The model under review builds one solid part; all positions refer to its coordinate system, in mm. Face numbers are marked on the shaded views. A direction names the side the tool comes from. Give positions to 0.01 mm unless a question says otherwise; leave off trailing zeros. Write each loop counter-clockwise with the first axis right and the second up, starting at its lowest first coordinate (ties: lowest second). Pieces come first, ordered by that corner, then holes. Notation, with made-up numbers: M -13.5,-36.75 L 27.5,-36.75 A10 cw 27.5,-18.75 Z; hole C 65,40.5 d9. An arc over 180 degrees is marked long. Write item = value, one per line. Start each with the question number.
Autodesk Inventor part; units mm, degrees
ref_plane "YZ Plane" through (0, 0, 0) normal (1, 0, 0) x (0, 1, 0)
ref_plane "XZ Plane" through (0, 0, 0) normal (0, 1, 0) x (-1, 0, 0)
ref_plane "XY Plane" through (0, 0, 0) normal (0, 0, 1) x (1, 0, 0)
sketch "スケッチ1" plane through (0, 0, 0) normal (0, 0, 1) x (1, 0, 0)
  line L0 (-32.5, -17.075) -> (32.5, -17.075)
  line L1 (32.5, -17.075) -> (32.5, 17.075)
  line L2 (32.5, 17.075) -> (-32.5, 17.075)
  line L3 (-32.5, 17.075) -> (-32.5, -17.075)
  line L4 (-32.5, -17.075) -> (32.5, 17.075) construction
  line L5 (32.5, -17.075) -> (-32.5, 17.075) construction
  point P0 (0, 0)
  dimension "d0" = 65
  dimension "d1" = 34.15
ref_plane "作業平面2" through (0, 0, -11.7) normal (0, 0, -1) x (-1, 0, 0)
ref_plane "作業平面1" through (35.75, -19.2175, -13.7) normal (0, 1, 0) x (-1, 0, 0)
sketch "スケッチ3" plane through (35.75, -19.2175, -13.7) normal (0, 1, 0) x (-1, 0, 0)
  line L0 (71.5, 0) -> (0, 0)
  line L1 (0, 0) -> (71.5, 0)
  line L2 (71.5, 0) -> (71.5, 20)
  line L3 (71.5, 20) -> (0, 20)
  line L4 (0, 20) -> (0, 0)
  line L5 (71.5, 1) -> (0, 1)
  point P0 (35.75, 13.7)
  dimension "d6" = 20
  dimension "d10" = 1
extrude "押し出し3" add sketch "スケッチ3" against normal blind 2
sketch "スケッチ4" plane through (35.75, -19.2175, -13.7) normal (0, 1, 0) x (1, 0, 0)
  line L0 (0, 0) -> (-71.5, 0)
  line L1 (0, -1) -> (-71.5, -1)
  line L2 (0, 0) -> (-71.5, 0)
  line L3 (-71.5, 0) -> (-71.5, -1)
  line L4 (-71.5, -1) -> (0, -1)
  line L5 (0, -1) -> (0, 0)
  point P0 (-35.75, -13.7)
extrude "押し出し4" add sketch "スケッチ4" along normal blind 38
sketch "スケッチ5" plane through (35.75, -19.2175, -13.7) normal (0, 1, 0) x (1, 0, 0)
  line L0 (0, 0) -> (0, -20)
  line L1 (0, -10) -> (-71.5, -10.5)
  line L2 (-71.5, -1) -> (-71.5, -20)
  point P0 (-35.75, -13.7)
  point P1 (-7, -10.049)
  point P2 (-20, -10.1399)
  point P3 (-33, -10.2308)
  point P4 (-46, -10.3217)
  point P5 (-59, -10.4126)
  dimension "d13" = 71.5
  dimension "d14" = 7
  dimension "d15" = 13
  dimension "d16" = 13
  dimension "d17" = 13
  dimension "d18" = 13
hole "穴1" at (28.75, -19.2175, -3.651) at (15.75, -19.2175, -3.5601) at (2.75, -19.2175, -3.4692) at (-10.25, -19.2175, -3.3783) at (-23.25, -19.2175, -3.2874) direction (0, -1, 0) diameter 3 depth 2 tip angle 118
sketch "スケッチ6" plane through (35.75, -21.2175, -13.7) normal (0, 0, -1) x (-1, 0, 0)
  line L0 (0, 2) -> (0, 40)
  line L1 (0, 0) -> (71.5, 0)
  line L2 (0, 40) -> (71.5, 40)
  line L3 (64, 7.25) -> (7.5, 7.25)
  line L4 (7.5, 7.25) -> (7.5, 32.75)
  line L5 (7.5, 32.75) -> (64, 32.75)
  line L6 (64, 32.75) -> (64, 7.25)
  line L7 (64, 7.25) -> (7.5, 32.75) construction
  line L8 (7.5, 7.25) -> (64, 32.75) construction
  point P0 (35.75, 21.2175)
  point P1 (35.75, 20)
  dimension "d26" = 56.5
  dimension "d27" = 25.5
hole "穴2" at (28.25, 11.5325, -13.7) at (28.25, -13.9675, -13.7) at (-28.25, 11.5325, -13.7) at (-28.25, -13.9675, -13.7) direction (0, 0, 1) diameter 2 depth 2 tip angle 118
properties part number "avhzy_maunt"
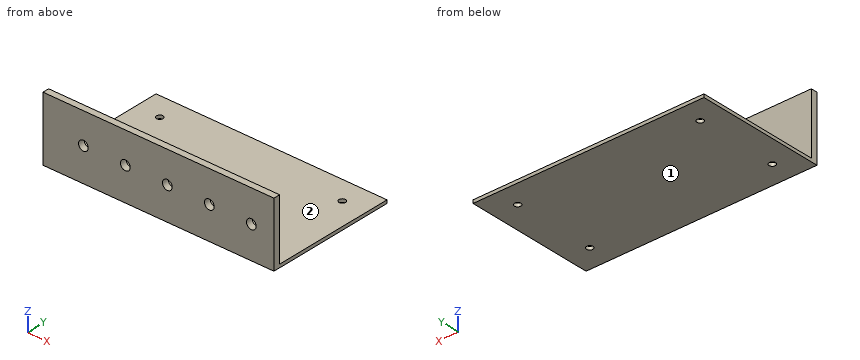
Item 1: To check wall thickness, follow probe 1 along Y at (x, z) = (28.25, -13.4); probe 2 along Y at (x, z) = (-1, 4); probe 3 along Z at (x, y) = (12, -16.5). State the ranges of each line that lie inside material, in increasing order. Write a range as [from, to].
Item 2: Clearance check with flat-ended pins moving along their axes: P1, Ø2.5, axis at x = 28.75, z = -3.651, coming from the +Y side; P2, Ø4, axis at x = 15.75, z = -3.56, coming from the +Y side; P3, Ø2.5, axis at x = -28.25, y = -13.97, coming from the +Z side. State where each tip first meets the part, or that it passes through.
Item 3: We need section C-C, the plane z = -6.5. Write out the cut boundary in (x, y), and give its area (3 significant figures).
Item 4: We need section D-D, the plane x = -12.5. Write out the cut boundary in (y, z).
Item 5: We need section A-A, the plane x = -28.25. Write out the cut boundary in (y, z).
Item 6: For the marked faces 1 and 2, list the 3-axis set-ups (+Z, -Z, +X, -X, +Y, -Y) from which the entire face can be reached by the end or side of a thin tool; tool diameter is ignored.
Item 7: We need section B-B, the plane x = 2. Write out the cut boundary in (y, z), and give its area (3 significant figures).
Worked out:
q1.probe_1 = [-21.22, -14.97], [-12.97, 10.53], [12.53, 18.78]
q1.probe_2 = [-21.22, -19.22]
q1.probe_3 = [-13.7, -12.7]
q2.P1 = through
q2.P2 = -19.22
q2.P3 = -12.7
q3.outline = M -35.75,-21.22 L 35.75,-21.22 L 35.75,-19.22 L -35.75,-19.22 Z
q3.area = 143 mm²
q4.outline = M -21.22,-13.7 L 18.78,-13.7 L 18.78,-12.7 L -19.22,-12.7 L -19.22,6.3 L -21.22,6.3 Z
q5.outline = M -21.22,-13.7 L -14.97,-13.7 L -14.97,-12.7 L -19.22,-12.7 L -19.22,6.3 L -21.22,6.3 Z; M -12.97,-13.7 L 10.53,-13.7 L 10.53,-12.7 L -12.97,-12.7 Z; M 12.53,-13.7 L 18.78,-13.7 L 18.78,-12.7 L 12.53,-12.7 Z
q6.face_1 = -Z, +X, -X, +Y, -Y
q6.face_2 = +Z, +X, -X, +Y
q7.outline = M -21.22,-13.7 L 18.78,-13.7 L 18.78,-12.7 L -19.22,-12.7 L -19.22,-4.77 L -21.22,-4.77 Z; M -21.22,-2.17 L -19.22,-2.17 L -19.22,6.3 L -21.22,6.3 Z
q7.area = 72.8 mm²
